Part model, mm, in its own coordinate system. A direction names the side the tool comes from. Give positions to 0.01 mm unless a question says otherwise; leave off trailing zeros. Write each loop counter-clockwise with the first axis right and the second up, starting at its lowest first coordinate (ties: lowest second). Pieces come first, ordered by that corner, then holes.
```python
from build123d import *

# Parameters (mm, degrees)
SKETCH1_R                       = 1.15
BOSS_EXTRUDE1_DEPTH             = 4
SKETCH2_W                       = 3.7
SKETCH2_H                       = 3.7
BOSS_EXTRUDE2_DEPTH             = 3.7
FILLET1_R                       = 0.5
SKETCH3_R                       = 1.25
BOSS_EXTRUDE3_DEPTH             = 3
FILLET2_R                       = 0.7
SKETCH4_R                       = 0.85
BOSS_EXTRUDE4_DEPTH             = 2.5
BOSS_EXTRUDE4_DIRECTION_2_REACH = 12.373
SKETCH5_R                       = 0.65
BOSS_EXTRUDE5_DEPTH             = 65
SKETCH6_R                       = 1.5
BOSS_EXTRUDE6_DEPTH             = 3
SKETCH7_R                       = 2.5
BOSS_EXTRUDE7_DEPTH             = 11
SKETCH8_R                       = 1.5
BOSS_EXTRUDE8_DEPTH             = 13
FILLET3_R                       = 1
FILLET4_R                       = 0.5
FILLET5_R                       = 0.5


with BuildPart() as part:
    # Sketch1 → Boss-Extrude1 (new body)
    with BuildSketch(Plane.XY):
        Circle(SKETCH1_R)
    extrude(amount=BOSS_EXTRUDE1_DEPTH)

    # Sketch2 → Boss-Extrude2 (add)
    with BuildSketch(Plane.XY.offset(4)):
        Rectangle(SKETCH2_W, SKETCH2_H)
    extrude(amount=BOSS_EXTRUDE2_DEPTH)

    # Fillet1
    fillet1_edges = [part.edges().sort_by_distance(p)[0] for p in [
        (-1.85, 0, 4),
        (-1.85, 1.85, 5.85),
        (0, -1.85, 4),
        (-1.85, -1.85, 5.85),
        (1.85, 0, 4),
        (1.85, -1.85, 5.85),
        (0, 1.85, 4),
        (1.85, 1.85, 5.85),
        (-1.85, 0, 7.7),
        (0, -1.85, 7.7),
        (1.85, 0, 7.7),
        (0, 1.85, 7.7),
    ]]
    fillet(fillet1_edges, radius=FILLET1_R)

    # Sketch3 → Boss-Extrude3 (add)
    with BuildSketch(Plane(origin=(0, 1.85, 0), x_dir=(1, 0, 0), z_dir=(0, 1, 0))):
        with Locations((0, -5.85)):
            Circle(SKETCH3_R)
    extrude(amount=BOSS_EXTRUDE3_DEPTH)

    # Fillet2
    fillet2_edges = [part.edges().sort_by_distance(p)[0] for p in [
        (-1.25, 4.85, 5.85),
    ]]
    fillet(fillet2_edges, radius=FILLET2_R)

    # Sketch4 → Boss-Extrude4 (add)
    with BuildSketch(Plane(origin=(0, 4.85, 0), x_dir=(1, 0, 0), z_dir=(0, 1, 0))):
        with Locations(Location((0, -5.85, 0), (0, 0, 180))):
            Circle(SKETCH4_R)
    extrude(amount=BOSS_EXTRUDE4_DEPTH)

    # Sketch4 → Boss-Extrude4 direction 2 (add, up to next)
    with BuildSketch(Plane(origin=(0, 4.85, 0), x_dir=(1, 0, 0), z_dir=(0, 1, 0)), mode=Mode.PRIVATE) as boss_extrude4_direction_2_sk1:
        with Locations(Location((0, -5.85, 0), (0, 0, 180))):
            Circle(SKETCH4_R)
    boss_extrude4_direction_2_tool1 = extrude(boss_extrude4_direction_2_sk1.sketch, amount=-BOSS_EXTRUDE4_DIRECTION_2_REACH, mode=Mode.PRIVATE) - part.part
    add(boss_extrude4_direction_2_tool1.solids().sort_by_distance((0, 4.85, 5.85))[0])

    # Sketch5 → Boss-Extrude5 (add)
    with BuildSketch(Plane(origin=(0, 7.35, 0), x_dir=(1, 0, 0), z_dir=(0, 1, 0))):
        with Locations(Location((0, -5.85, 0), (0, 0, 180))):
            Circle(SKETCH5_R)
    extrude(amount=BOSS_EXTRUDE5_DEPTH)

    # Sketch6 → Boss-Extrude6 (add)
    with BuildSketch(Plane(origin=(0, 72.35, 0), x_dir=(1, 0, 0), z_dir=(0, 1, 0))):
        with Locations(Location((0, -5.85, 0), (0, 0, 180))):
            Circle(SKETCH6_R)
    extrude(amount=BOSS_EXTRUDE6_DEPTH)

    # Sketch7 → Boss-Extrude7 (add)
    with BuildSketch(Plane(origin=(0, 75.35, 0), x_dir=(1, 0, 0), z_dir=(0, 1, 0))):
        with Locations(Location((0, -5.85, 0), (0, 0, 180))):
            Circle(SKETCH7_R)
    extrude(amount=BOSS_EXTRUDE7_DEPTH)

    # Sketch8 → Boss-Extrude8 (add)
    with BuildSketch(Plane(origin=(0, 86.35, 0), x_dir=(1, 0, 0), z_dir=(0, 1, 0))):
        with Locations(Location((0, -5.85, 0), (0, 0, 180))):
            Circle(SKETCH8_R)
    extrude(amount=BOSS_EXTRUDE8_DEPTH)

    # Fillet3
    fillet3_edges = [part.edges().sort_by_distance(p)[0] for p in [
        (2.5, 86.35, 5.85),
    ]]
    fillet(fillet3_edges, radius=FILLET3_R - 0.0001)  # a hair under: the kernel refuses the full size

    # Fillet4
    fillet4_edges = [part.edges().sort_by_distance(p)[0] for p in [
        (2.5, 75.35, 5.85),
    ]]
    fillet(fillet4_edges, radius=FILLET4_R)

    # Fillet5
    fillet5_edges = [part.edges().sort_by_distance(p)[0] for p in [
        (1.5, 75.35, 5.85),
    ]]
    fillet(fillet5_edges, radius=FILLET5_R - 0.0001)  # a hair under: the kernel refuses the full size


solid = part.part
```
1) Two-plate mould, pull along Y, no slides. Class faces 1 (the face through (0, 99.35, 6)), 2 (the face through (-1, 72.35, 6)), 3 (the face through (-1.85, 0, 6)): +Y half, -Y half, draft (parallel to the pull), parting line (faces both ways), or undercut.
Answers follow:
face 1: +Y half
face 2: undercut
face 3: draft
2) Pin check, flat tips, straight feed: pin 1 Ø0.8 at (x, y) = (0.5, -0.5) entering from +Z; pin 2 Ø2 at (y, z) = (0.5, 6) entering from -X; pin 3 Ø2 at (x, y) = (-0.5, 22) entering from -Z. Stop position of each tip, or through.
Answers follow:
pin 1: stops at z = 7.7
pin 2: stops at x = -1.85
pin 3: stops at z = 5.2
3) 3-axis set-ups, long thin cutter, end or side, ignore diameter. For faces 4 (the face through (0.325, 92.759, 4.386)), 5 (the face through (0, 0, 7.7)), 6 (the face through (1.85, 0, 6)), 7 (the face through (-0.91, -0.7, 1.97)), 8 (the face through (0.325, 73.583, 4.386)): which of +Z, -Z, +X, -X, +Y, -Y reach the whole face in a straight line?
Answers follow:
face 4: +Y
face 5: +Z, +X, -X, -Y
face 6: +Z, -Z, +X, -Y
face 7: -Z
face 8: none
4) Wall check: L1, parallel to Y at x = -0.6, z = 5.5; L2, parallel to Y at x = -0.55, z = 4.5; L3, parallel to X at y = 55.5, z = 6. Give the ranges that are in metal, low to high.
Answers follow:
L1: y = -1.85 to 7.35, 72.35 to 99.35
L2: y = -1.85 to 1.85, 72.35 to 99.35
L3: x = -0.63 to 0.63
5) Saw through at C-C, the plane y = 33. Write the cut outline in (x, z), then the cut area to 3 significant figures.
Answers follow:
outline: circle Ø1.3 at (0, 5.85)
area: 1.33 mm2
6) Saw through at B-B, the plane z = 1. Write the cut outline in (x, y).
Answers follow:
outline: circle Ø2.3 at (0, 0)
7) Saw through at A-A, the plane y = 0. Write the cut outline in (x, z).
Answers follow:
outline: (-1.85, 4.5) arc R0.5 ccw to (-1.35, 4) - (-1.15, 4) - (-1.15, 0) - (1.15, 0) - (1.15, 4) - (1.35, 4) arc R0.5 ccw to (1.85, 4.5) - (1.85, 7.2) arc R0.5 ccw to (1.35, 7.7) - (-1.35, 7.7) arc R0.5 ccw to (-1.85, 7.2) - close
